Could you check a few things on this drawing? It's one solid part, dimensions in mm from its lowest x, y, z. Round coordinates to 2 decimals unless told otherwise and drop trailing zeros. Loops run counter-clockwise (first coordinate to the right, second up) from the corner with the lowest first, then second, coordinate; pieces in that order, holes last. Notation, with made-up numbers: M 24,-30.75 L 44,-30.75 A21 ccw 44,-21.75 Z; hole C 52,7.5 d1. An arc over 180 degrees is marked long. Write item = value, one per line. Start each with the question number.
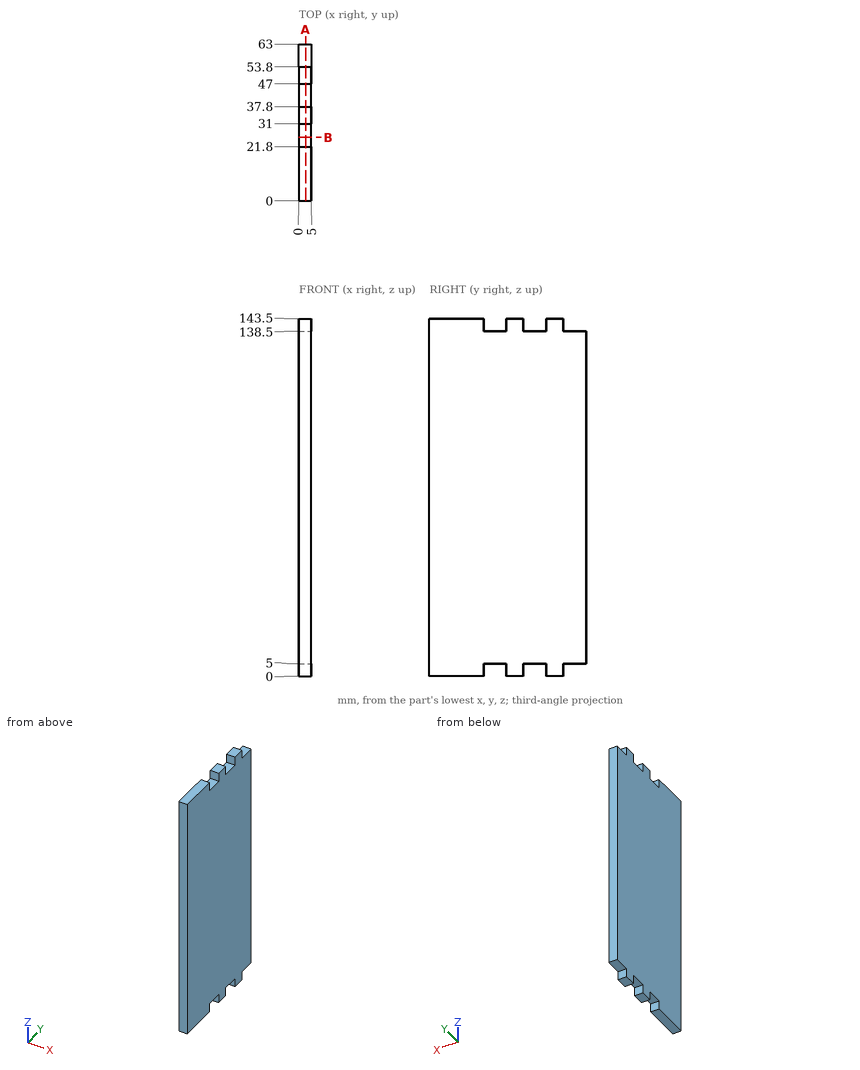
Item 1: Will these pins go through, and if not, where does the flat tip stop? pin 1 Ø1.5 at (x, y) = (2, 57.5) entering from +Z; pin 2 Ø1.5 at (x, z) = (3.5, 142) entering from +Y; pin 3 Ø1.5 at (x, y) = (1.5, 42) entering from -Z.
Item 2: Please list where this line runs through material, in increasing order: line 1 (Z direction, x = 2, y = 22.5). Write a range as [from, to].
Item 3: I want a section at B-B, the plane y = 25.5. List the corners of the cut face in (x, z) for me, then the cut area to 4 significant figures.
Item 4: I want a section at A-A, the plane x = 2.7. List the corners of the cut face in (y, z) for me, then the cut area to 3 significant figures.
Worked out:
q1.pin_1 = 138.5
q1.pin_2 = 53.8
q1.pin_3 = 5
q2.line_1 = [5, 138.5]
q3.outline = M 0,5 L 5,5 L 5,138.5 L 0,138.5 Z
q3.area = 667.5 mm2
q4.outline = M 0,0 L 21.8,0 L 21.8,5 L 31,5 L 31,0 L 37.8,0 L 37.8,5 L 47,5 L 47,0 L 53.8,0 L 53.8,5 L 63,5 L 63,138.5 L 53.8,138.5 L 53.8,143.5 L 47,143.5 L 47,138.5 L 37.8,138.5 L 37.8,143.5 L 31,143.5 L 31,138.5 L 21.8,138.5 L 21.8,143.5 L 0,143.5 Z
q4.area = 8,760 mm2
